from build123d import *

# Parameters (mm, degrees)
SKETCH1_R           = 90
BOSS_EXTRUDE1_DEPTH = 5
CUT_EXTRUDE1_DEPTH  = 44
SKETCH3_R           = 3
CUT_EXTRUDE2_DEPTH  = 129
FILLET1_R           = 20


with BuildPart() as part:
    # Sketch1 → Boss-Extrude1 (new body)
    with BuildSketch(Plane.XY):
        Circle(SKETCH1_R)
    extrude(amount=BOSS_EXTRUDE1_DEPTH)

    # Sketch2 → Cut-Extrude1 (cut)
    with BuildSketch(Plane.XY.offset(5)):
        with BuildLine():
            Line((69.768328483, -87.081626915), (45.971435375, -105.349299959))
            Line((45.971435375, -105.349299959), (-14.920808105, -26.026322935))
            ThreePointArc((-14.920808105, -26.026322935), (-2.321306127, 29.91005747), (18.757736535, -23.412546211))
            Line((18.757736535, -23.412546211), (69.768328483, -87.081626915))
        make_face()
    extrude(amount=-CUT_EXTRUDE1_DEPTH, mode=Mode.SUBTRACT)

    # Sketch3 → Cut-Extrude2 (cut)
    with BuildSketch(Plane.XY.offset(5)):
        with Locations((62.5, 0)):
            Circle(SKETCH3_R)
        with Locations((44.194173824, -44.194173824)):
            Circle(SKETCH3_R)
        with Locations((0, -62.5)):
            Circle(SKETCH3_R)
        with Locations((-44.194173824, -44.194173824)):
            Circle(SKETCH3_R)
        with Locations((-62.5, 0)):
            Circle(SKETCH3_R)
        with Locations((-44.194173824, 44.194173824)):
            Circle(SKETCH3_R)
        with Locations((0, 62.5)):
            Circle(SKETCH3_R)
        with Locations((44.194173824, 44.194173824)):
            Circle(SKETCH3_R)
    extrude(amount=-CUT_EXTRUDE2_DEPTH, mode=Mode.SUBTRACT)

    # Fillet1
    fillet1_edges = [part.edges().sort_by_distance(p)[0] for p in [
        (-14.920808105, -26.026322935, 2.5),
        (56.273209604, -70.237638634, 2.5),
        (18.757736535, -23.412546211, 2.5),
        (30.18651872, -84.786638615, 2.5),
    ]]
    fillet(fillet1_edges, radius=FILLET1_R)


solid = part.part
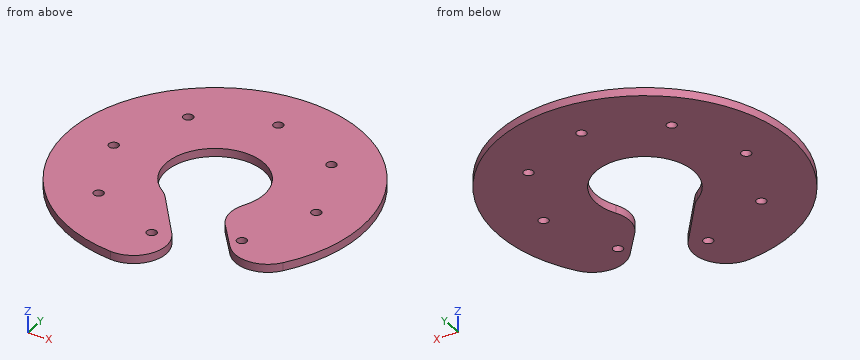
Check sheet for the modelled part. Datum: model origin and axes. Units: mm. Round coordinates to 2 decimals unless told otherwise and drop trailing zeros. Write each loop counter-clockwise with the first axis right and the second up, starting at its lowest first coordinate (ties: lowest second). Pieces come first, ordered by that corner, then holes. Notation, with made-up numbers: (31, -6) - (56, -6) arc R15 cw to (56, -2) - close; hole circle Ø4 at (32, -6). An arc over 180 degrees is marked (long way). Return JSON: item names as keys, results as strings.
Q1. Scan lines: L1, parallel to X at y = -52, z = 4.3; L2, parallel to Y at x = 0, z = 1.1; L3, parallel to X at y = -10, z = 4.4. Record each from-to range of solid material in increasing order. Write a range as from..to.
Returned:
{"L1": "x = -73.46..5.02, 41.66..73.44", "L2": "y = -88.56..-65.5, -59.5..-45.46, 30..59.5, 65.5..90", "L3": "x = -89.44..-28.28, 28.28..89.44"}
Q2. Cross-section at D-D (x = 0). Record the boundary of the cut face in (y, z).
Returned:
{"outline": "(-88.56, 0) - (-65.5, 0) - (-65.5, 5) - (-88.56, 5) - close; (-59.5, 0) - (-45.46, 0) - (-45.46, 5) - (-59.5, 5) - close; (30, 0) - (59.5, 0) - (59.5, 5) - (30, 5) - close; (65.5, 0) - (90, 0) - (90, 5) - (65.5, 5) - close"}
Q3. Cross-section at B-B (x = 62.5). Record the boundary of the cut face in (y, z).
Returned:
{"outline": "(-59.23, 0) - (-3, 0) - (-3, 5) - (-59.23, 5) - close; (3, 0) - (64.76, 0) - (64.76, 5) - (3, 5) - close"}
Q4. Cross-section at C-C (z = 1.55). Give the number of separate pieces and of enclosed holes in the cut face, then the cut area to 3 significant figures.
Returned:
{"separate pieces": "1", "enclosed holes": "8", "area": "20,100 mm²"}
Q5. Depth check by flat-ended pin: P1, Ø3.5, axis at x = -44.19, y = -44.19, coming from the +Z side; P2, Ø6, axis at x = -53.5, y = -59, coming from the -Z side; P3, Ø3, axis at x = -13, z = 4.5, coming from the +Y side; P4, Ø2, axis at y = -46.5, z = 1, coming from the +X side. Enter the tip coordinate at first touch or a pass-through.
Returned:
{"P1": "passes through", "P2": "stops at z = 0", "P3": "stops at y = 89.26", "P4": "stops at x = 77.65"}
Q6. Cross-section at A-A (y = 0). Record the boundary of the cut face in (x, z), then the cut area to 3 significant figures.
Returned:
{"outline": "(-90, 0) - (-65.5, 0) - (-65.5, 5) - (-90, 5) - close; (-59.5, 0) - (-30, 0) - (-30, 5) - (-59.5, 5) - close; (30, 0) - (59.5, 0) - (59.5, 5) - (30, 5) - close; (65.5, 0) - (90, 0) - (90, 5) - (65.5, 5) - close", "area": "540 mm²"}
